from build123d import *

# Parameters (mm, degrees)
SKETCH1_R           = 30
BOSS_EXTRUDE1_DEPTH = 10
SKETCH2_W           = 70.710678118
SKETCH2_H           = 80
BOSS_EXTRUDE2_DEPTH = 200
SKETCH3_R           = 10
CUT_EXTRUDE1_DEPTH  = 150
SHELL1_START        = 12
SHELL1_OUTLINE_W    = 66.710678118
SHELL1_OUTLINE_H    = 76
SHELL1_OUTLINE_R    = 12
SHELL1_DEPTH        = 196
SHELL1_START_2      = 2
SHELL1_2_OUTLINE_R  = 28
SHELL1_2_DEPTH      = 56
FILLET1_R           = 5


# Read off the part's stored shape, not the designer's step: Shell1
with BuildPart() as part:
    # Sketch1 → Boss-Extrude1 (new body)
    with BuildSketch(Plane.XY):
        Circle(SKETCH1_R)
    extrude(amount=BOSS_EXTRUDE1_DEPTH)

    # Sketch2 → Boss-Extrude2 (add)
    with BuildSketch(Plane.XY.offset(10)):
        Rectangle(SKETCH2_W, SKETCH2_H)
    extrude(amount=BOSS_EXTRUDE2_DEPTH)

    # Sketch3 → Cut-Extrude1 (cut)
    with BuildSketch(Plane.XY.offset(210)):
        Circle(SKETCH3_R)
    extrude(amount=-CUT_EXTRUDE1_DEPTH, mode=Mode.SUBTRACT)

    # Shell1 outline → Shell1 (cut)
    with BuildSketch(Plane.XY.offset(SHELL1_START)):
        Rectangle(SHELL1_OUTLINE_W, SHELL1_OUTLINE_H)
        Circle(SHELL1_OUTLINE_R, mode=Mode.SUBTRACT)
    extrude(amount=SHELL1_DEPTH, mode=Mode.SUBTRACT)

    # Shell1 2 outline → Shell1 2 (cut)
    with BuildSketch(Plane.XY.offset(SHELL1_START_2)):
        Circle(SHELL1_2_OUTLINE_R)
    extrude(amount=SHELL1_2_DEPTH, mode=Mode.SUBTRACT)

    # Fillet1
    fillet1_edges = [part.edges().sort_by_distance(p)[0] for p in [
        (-35.355339059, 40, 110),
        (-35.355339059, -40, 110),
        (35.355339059, -40, 110),
        (35.355339059, 40, 110),
    ]]
    fillet(fillet1_edges, radius=FILLET1_R)


solid = part.part
Geometry: final body of the model. Coordinates: model frame, mm. A direction names the side the tool comes from. Coordinates: 2 decimals unless noted, no trailing zeros. Loops run counter-clockwise (first coordinate to the right, second up) from the corner with the lowest first, then second, coordinate; pieces in that order, holes last. Notation, with made-up numbers: (54.5, -26) - (87.5, -26) arc R22 cw to (87.5, -9) - close; hole circle Ø10 at (-38.5, -34). An arc over 180 degrees is marked (long way). One line per question, with ' | ' between items. Start each with the question number.
(1) Cut plane C-C on y = 0. Output: boundary loops of the cut face in (x, z), and give its area (3 significant figures).
(2) Draft query along Z for faces 1 (the flat face through (-33.355, -1, 109)), 2 (the flat face through (-24.1, 18.3, 10)), 3 (the flat face through (7, 9, 210)). Return one class per face: +Z half, -Z half, draft (parallel to the pull), parting line (faces both ways), or undercut.
(3) Cut plane B-B on x = 0. Output: boundary loops of the cut face in (y, z), and give its area (3 significant figures).
(4) Reachability of faces 4 (the flat face through (0, -38, 109)), 5 (the cylindrical face through (-2.17, -9.76, 136.05)), 6 (the cylindrical face through (-29.97, 1.32, 4.93)), 7 (the cylindrical face through (33.852, -38.574, 111.4)) from +Z, -Z, +X, -X, +Y, -Y: full face, straight path, thin tool, end or side. Return the list, or none.
(5) First-contact query: pin 1 (1.5 mm diameter, centred on x = -15, y = 25, fed in from -Z); pin 2 (6 mm diameter, centred on x = -3.5, y = -2.5, fed in from +Z). Flat tips, straight axial feed; report the tip coordinate or a pass-through.
(6) Cut plane D-D on z = 44.5. Output: boundary loops of the cut face in (x, y), and give its area (3 significant figures).
(7) Ray query, L1, parallel to Y at x = 0, z = 128; L2, parallel to X at y = -30, z = 182; L3, parallel to Y at x = 20.5, z = 149. Return the intervals inside material, ascending. Write a range as from..to.
(8) Cut plane A-A on z = 107. Output: boundary loops of the cut face in (x, y), and give its area (3 significant figures).
Here are the results:
1) outline: (-35.36, 10) - (-30, 10) - (-30, 0) - (30, 0) - (30, 10) - (35.36, 10) - (35.36, 210) - (10, 210) - (10, 60) - (-10, 60) - (-10, 210) - (-35.36, 210) - close; hole (-33.36, 12) - (-28, 12) - (-28, 2) - (28, 2) - (28, 12) - (33.36, 12) - (33.36, 208) - (12, 208) - (12, 58) - (-12, 58) - (-12, 208) - (-33.36, 208) - close | area: 1,710 mm²
2) face 1: undercut | face 2: -Z half | face 3: +Z half
3) outline: (-40, 10) - (-30, 10) - (-30, 0) - (30, 0) - (30, 10) - (40, 10) - (40, 210) - (10, 210) - (10, 60) - (-10, 60) - (-10, 210) - (-40, 210) - close; hole (-38, 12) - (-28, 12) - (-28, 2) - (28, 2) - (28, 12) - (38, 12) - (38, 208) - (12, 208) - (12, 58) - (-12, 58) - (-12, 208) - (-38, 208) - close | area: 1,740 mm²
4) face 4: none | face 5: +Z | face 6: -Z | face 7: +Z, -Z, +X, -Y
5) pin 1: z = 0 | pin 2: z = 60
6) outline: (-35.36, -35) arc R5 ccw to (-30.36, -40) - (30.36, -40) arc R5 ccw to (35.36, -35) - (35.36, 35) arc R5 ccw to (30.36, 40) - (-30.36, 40) arc R5 ccw to (-35.36, 35) - close; hole (-33.36, -38) - (33.36, -38) - (33.36, 38) - (-33.36, 38) - close | area: 565 mm²
7) L1: -40..-38, -12..-10, 10..12, 38..40 | L2: -35.36..-33.36, 33.36..35.36 | L3: -40..-38, 38..40
8) outline: (-35.36, -35) arc R5 ccw to (-30.36, -40) - (30.36, -40) arc R5 ccw to (35.36, -35) - (35.36, 35) arc R5 ccw to (30.36, 40) - (-30.36, 40) arc R5 ccw to (-35.36, 35) - close; circle Ø24 at (0, 0); hole (-33.36, -38) - (33.36, -38) - (33.36, 38) - (-33.36, 38) - close; hole circle Ø20 at (0, 0) | area: 704 mm²
